Build history of the part. All positions in model axes, mm. Face numbers are marked on the shaded views. A direction names the side the tool comes from. Give positions to 0.01 mm unless a question says otherwise; leave off trailing zeros. Order: outer loops, then holes, each group sorted by start corner. A loop starts at its lowest first (then second) coordinate and runs counter-clockwise, first axis right, second up. Notation, with made-up numbers: (-37, 73) - (1, 73) arc R7 ccw to (1, 82) - close; hole circle Ø9 at (32.25, -37.75). An arc over 180 degrees is marked (long way). Answer in a Markdown table with one row per item.
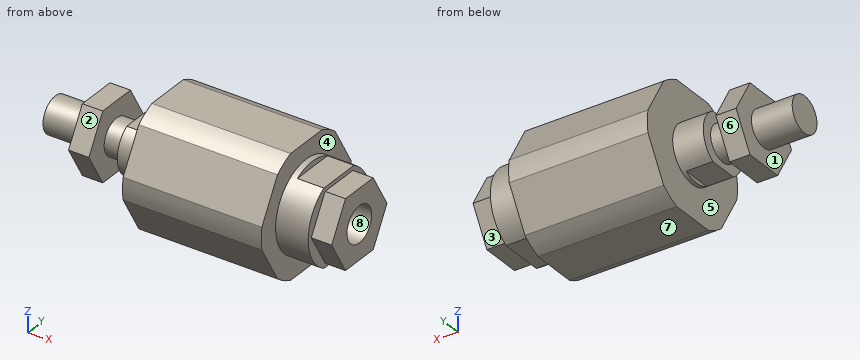
```python
from build123d import *

# Parameters (mm, degrees)
OUTSIDE_FLATSS_OUTSIDE_W = 50.588
OUTSIDE_FLATSS_OUTSIDE_H = 50.588
OUTSIDE_FLATS_DEPTH      = 74.090697082
FRONT_NUT_DEPTH          = 5
FRONT_START              = -6.5
FRONT_FLATS_DEPTH        = 6.5
REAR_FLATS_DEPTH         = 6.5
REAR_START               = 5
REAR_NUT_SK_R            = 4.4
REAR_NUT_DEPTH           = 5


with BuildPart() as part:
    # Bodies → Body (revolve)
    with BuildSketch(Plane.XY, mode=Mode.PRIVATE) as body_sk:
        Polygon((-69.5, 4.4), (-49.5, 4.4), (-49.5, 7), (-42, 7), (-42, 16), (-8, 16), (-8, 10.9), (0, 10.9), (0, 4.4), (-23, 4.4), (-23, 0), (-69.5, 0), align=None)
    revolve(body_sk.sketch.rotate(Axis((0, 0, 0), (-1, 0, 0)), 90), axis=Axis((0, 0, 0), (-1, 0, 0)))

    # Outside Flatss outside → Outside Flats (cut, through all)
    with BuildSketch(Plane.ZY.offset(69.5)):
        Rectangle(OUTSIDE_FLATSS_OUTSIDE_W, OUTSIDE_FLATSS_OUTSIDE_H)
        Polygon((0, 17.320508076), (15, 8.660254038), (15, -8.660254038), (0, -17.320508076), (-15, -8.660254038), (-15, 8.660254038), align=None, mode=Mode.SUBTRACT)
    extrude(amount=-OUTSIDE_FLATS_DEPTH, mode=Mode.SUBTRACT)

    # Front Nuts → Front Nut (add)
    with BuildSketch(Plane.ZY.offset(59.5)):
        Polygon((0, 9.814954576), (8.5, 4.907477288), (8.5, -4.907477288), (0, -9.814954576), (-8.5, -4.907477288), (-8.5, 4.907477288), align=None)
    extrude(amount=-FRONT_NUT_DEPTH)

    # Front Flatss → Front Flats (cut)
    with BuildSketch(Plane.ZY.offset(49.5).offset(FRONT_START)):
        with BuildLine():
            Line((-6, 3.605551275), (-6, -3.605551275))
            ThreePointArc((-6, -3.605551275), (-7, 0), (-6, 3.605551275))
        make_face()
        with BuildLine():
            Line((6, 3.605551275), (6, -3.605551275))
            ThreePointArc((6, -3.605551275), (7, 0), (6, 3.605551275))
        make_face()
    extrude(amount=FRONT_FLATS_DEPTH, mode=Mode.SUBTRACT)

    # Rear Flatss → Rear Flats (cut)
    with BuildSketch(Plane(origin=(0, 0, 0), x_dir=(0, 0, -1), z_dir=(1, 0, 0))):
        with BuildLine():
            Line((-9.5, 5.344155686), (-9.5, -5.344155686))
            ThreePointArc((-9.5, -5.344155686), (-10.9, 0), (-9.5, 5.344155686))
        make_face()
        with BuildLine():
            Line((9.5, 5.344155686), (9.5, -5.344155686))
            ThreePointArc((9.5, -5.344155686), (10.9, 0), (9.5, 5.344155686))
        make_face()
    extrude(amount=-REAR_FLATS_DEPTH, mode=Mode.SUBTRACT)

    # Rear Nut sk → Rear Nut (add)
    with BuildSketch(Plane(origin=(0, 0, 0), x_dir=(0, 0, -1), z_dir=(1, 0, 0)).offset(REAR_START)):
        Polygon((8.5, 4.907477288), (0, 9.814954576), (-8.5, 4.907477288), (-8.5, -4.907477288), (0, -9.814954576), (8.5, -4.907477288), align=None)
        Circle(REAR_NUT_SK_R, mode=Mode.SUBTRACT)
    extrude(amount=-REAR_NUT_DEPTH)


solid = part.part
```
1. Two-plate mould, pull along Y, no slides. Class the marked faces 6, 7 and 8: +Y half, -Y half, draft (parallel to the pull), parting line (faces both ways), or undercut.
Check result:
| item | result |
|---|---|
| face 6 | +Y half |
| face 7 | draft |
| face 8 | undercut |
2. Drop flat-ended pins along their axis: P1, Ø4, axis at x = -6.5, z = -11, coming from the +Y side; P2, Ø3, axis at y = 8, z = 0, coming from the -X side; P3, Ø5.5, axis at x = 3.5, y = -2, coming from the -Z side; P4, Ø5, axis at y = 2.5, z = -1.5, coming from the +X side. Give the stop position or say it passes through.
Check result:
| item | result |
|---|---|
| P1 | stops at y = 11.73 |
| P2 | stops at x = -59.5 |
| P3 | stops at z = -8.5 |
| P4 | stops at x = 5 |
3. Probe line 1 (Z direction, x = -9, y = 0); line 2 (Z direction, x = -4, y = 0); line 3 (X direction, y = -2, z = -5.75). List the from-to ranges inside material, lowest first.
Check result:
| item | result |
|---|---|
| line 1 | z = -15 to -4.4, 4.4 to 15 |
| line 2 | z = -9.5 to -4.4, 4.4 to 9.5 |
| line 3 | x = -59.5 to -54.5, -49.5 to 5 |
4. Cut at B-B on x = -56.5. Write the cut outline in (y, z), and give its area (3 significant figures).
Check result:
| item | result |
|---|---|
| outline | (-9.81, 0) - (-4.91, -8.5) - (4.91, -8.5) - (9.81, 0) - (4.91, 8.5) - (-4.91, 8.5) - close |
| area | 250 mm² |
5. Cut at A-A on y = -9. Write the cut outline in (x, z), and give its area (3 significant figures).
Check result:
| item | result |
|---|---|
| outline | (-59.5, -1.41) - (-54.5, -1.41) - (-54.5, 1.41) - (-59.5, 1.41) - close; (-42, -13.23) - (-8, -13.23) - (-8, -6.15) - (0, -6.15) - (0, -1.41) - (5, -1.41) - (5, 1.41) - (0, 1.41) - (0, 6.15) - (-8, 6.15) - (-8, 13.23) - (-42, 13.23) - close |
| area | 1,030 mm² |
6. Which spindle directions (+Z, -Z, +X, -X, +Y, -Y) get a long thin tool onto all of the face, cutting with end or side? Do the marked faces 1, 2, 3, 4 and 5. Say none if no direction does.
Check result:
| item | result |
|---|---|
| face 1 | -X |
| face 2 | +Z, -X, -Y |
| face 3 | -Z, +X, +Y |
| face 4 | +X |
| face 5 | none |
